The model under review builds one solid part; all positions refer to its coordinate system, in mm. A direction names the side the tool comes from. Coordinates: 2 decimals unless noted, no trailing zeros. Loops run counter-clockwise (first coordinate to the right, second up) from the corner with the lowest first, then second, coordinate; pieces in that order, holes last. Notation, with made-up numbers: M 66,42 L 87,42 A23 cw 87,65 Z; hole C 48.25,64.25 d6. An arc over 180 degrees is marked long. One line per item, written item: value.
```python
from build123d import *

# Parameters (mm, degrees)
SKETCH1_W          = 116.84
SKETCH1_H          = 6.223
SKETCH3_W          = 1.4224
SKETCH3_H          = 0.5588
CUT_EXTRUDE1_DEPTH = 1.5875


with BuildPart() as part:
    # Sketch1 → Revolve1 (revolve)
    with BuildSketch(Plane(origin=(0, 0, 0), x_dir=(0, 0, -1), z_dir=(1, 0, 0)), mode=Mode.PRIVATE) as revolve1_sk:
        with Locations((58.42, 3.1115)):
            Rectangle(SKETCH1_W, SKETCH1_H)
    revolve(revolve1_sk.sketch.rotate(Axis((0, 0, 0), (0, 0, 1)), 90), axis=Axis((0, 0, 0), (0, 0, 1)))

    # Sketch3 → Cut-Revolve1 (revolve, cut)
    with BuildSketch(Plane(origin=(0, 0, 0), x_dir=(0, 0, -1), z_dir=(1, 0, 0))):
        with Locations((1.7272, 6.223)):
            Rectangle(SKETCH3_W, SKETCH3_H)
        with Locations((61.5696, 6.223)):
            Rectangle(SKETCH3_W, SKETCH3_H)
        with Locations((20.2946, 6.223)):
            Rectangle(SKETCH3_W, SKETCH3_H)
        with Locations((115.1128, 6.223)):
            Rectangle(SKETCH3_W, SKETCH3_H)
    revolve(axis=Axis((0, 0, 0), (0, 0, 1)), mode=Mode.SUBTRACT)

    # Sketch4 → Cut-Extrude1 (cut)
    with BuildSketch(Plane(origin=(0, 6.223, 0), x_dir=(1, 0, 0), z_dir=(0, 1, 0))):
        with BuildLine():
            Line((-1.5875, 26.7335), (-1.5875, 58.6105))
            ThreePointArc((-1.5875, 58.6105), (0, 60.198), (1.5875, 58.6105))
            Line((1.5875, 58.6105), (1.5875, 26.7335))
            ThreePointArc((1.5875, 26.7335), (0, 25.146), (-1.5875, 26.7335))
        make_face()
    extrude(amount=-CUT_EXTRUDE1_DEPTH, mode=Mode.SUBTRACT)


solid = part.part
```
(1) Add section A-A on z = -91.5. State the section outline as (x, y) points, then the cut area to 3 significant figures.
Checks:
outline: C 0,0 d12.45
area: 122 mm^2
(2) To check wall thickness, follow L1, parallel to Z at x = -3, y = -5.25; L2, parallel to Z at x = 0, y = 4.75; L3, parallel to X at y = 0.25, z = -62. State the ranges of each line that lie inside material, in increasing order. Write a range as [from, to].
Checks:
L1: [-116.84, -115.82], [-114.4, -62.28], [-60.86, -21.01], [-19.58, -2.44], [-1.02, 0]
L2: [-116.84, -60.2], [-25.15, 0]
L3: [-5.94, 5.94]
(3) Add section B-B on z = -29. State the section outline as (x, y) points, then the cut area to 3 significant figures.
Checks:
outline: M -1.59,4.64 L -1.59,6.02 A6.22 ccw long 1.59,6.02 L 1.59,4.64 Z
area: 117 mm^2
(4) Draft analysis for pull direction X (two halves, no side actions). For faces 3 (the face through (0, 4.636, -43)), 4 (the face through (0, 0, 0)), 5 (the face through (-2.87, 5.52, -116.34)), state which applies: pulls with the +X half, pulls with the -X half, needs draft (parallel to the pull), parting line crosses it, or undercut.
Checks:
face 3: undercut
face 4: needs draft
face 5: parting line crosses it
(5) Tool access review of faces 1 (the face through (-1.785, 5.669, -1.737)), 2 (the face through (-2.87, 5.52, -0.52)): name each direction out of +Z, -Z, +X, -X, +Y, -Y from which nothing blocks a thin tool from reaching the whole face with its end or side.
Checks:
face 1: none
face 2: +Z, -Z
(6) Insertion check: pin 1 Ø5 at (x, z) = (2, -32.5) entering from +Y; pin 2 Ø2 at (x, z) = (-3, -63.5) entering from +Y; pin 3 Ø2 at (x, y) = (1.5, -1.5) entering from +Z; pin 4 Ø5 at (y, z) = (-4.5, -56.5) entering from -X. Each pin has a flat end and moves straight along its axis. Give the tip position at first contact, or say it passes through.
Checks:
pin 1: y = 6.02
pin 2: y = 5.89
pin 3: z = 0
pin 4: x = -5.89
